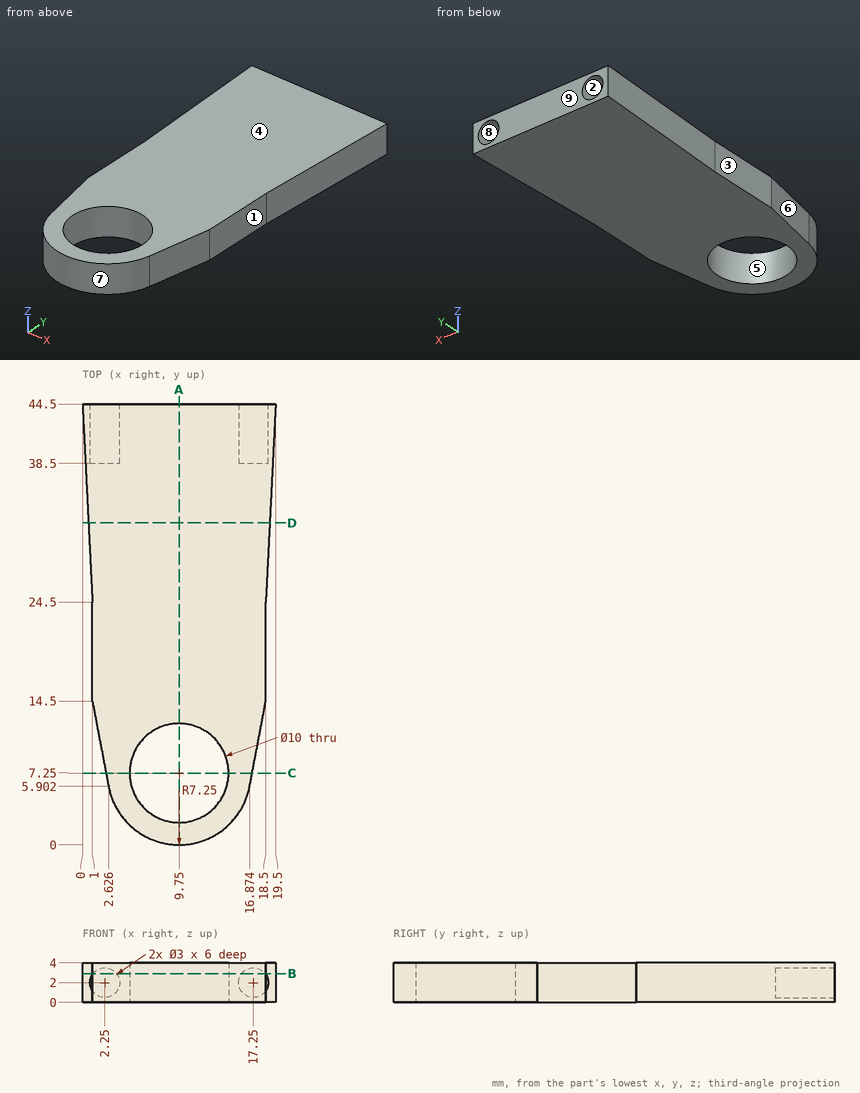
Geometry check sheet. Reference: drawing and pictorial views, mm from the part's lowest x, y, z. A direction names the side the tool comes from. Give positions to 0.01 mm unless a question says otherwise; leave off trailing zeros. Loops run counter-clockwise (first coordinate to the right, second up) from the corner with the lowest first, then second, coordinate; pieces in that order, holes last. Notation, with made-up numbers: M 65,23.25 L 121,23.25 A25 cw 121,61.25 Z; hole C -3,-10.5 d2. An arc over 180 degrees is marked long. One line per question, with ' | ' between items.
Item 1: Depth check by flat-ended pin: P1, Ø2, axis at y = 18, z = 1.5, coming from the -X side; P2, Ø1.2, axis at y = 18.5, z = 2.5, coming from the +X side; P3, Ø1.8, axis at x = 17.25, z = 2, coming from the +Y side. Enter the tip coordinate at first touch or a pass-through.
Completed:
P1: stops at x = 1 | P2: stops at x = 18.5 | P3: stops at y = 38.5
Item 2: Section check D-D, the plane y = 32.5. Record the cut outline in (x, z), plus the area to 3 significant figures.
Completed:
outline: M 0.6,0 L 18.9,0 L 18.9,4 L 0.6,4 Z | area: 73.2 mm^2
Item 3: Draft check along X on the marked faces 6, 7, 8 and 9. Enter one of: +X half, -X half, draft (parallel to the pull), parting line (faces both ways), or undercut.
Completed:
face 6: -X half | face 7: parting line | face 8: undercut | face 9: draft
Item 4: Tool access check on the marked faces 1, 2, 3, 4 and 5. Record the directions out of +Z, -Z, +X, -X, +Y, -Y that give a thin tool (end or side, any length) a straight path to the whole face; none if there is none.
Completed:
face 1: +Z, -Z, +X, -Y | face 2: +Y | face 3: +Z, -Z, -X, -Y | face 4: +Z, +X, -X, +Y, -Y | face 5: +Z, -Z
Item 5: Thickness scan on line 1 (Z direction, x = 2.25, y = 41.15); line 2 (Y direction, x = 9.5, z = 0.55) (1 decimal); line 3 (Y direction, x = 7, z = 1.65) (1 decimal). Record the ranges inside material, lowest first. Write a range as [from, to].
Completed:
line 1: z = [0, 0.5], [3.5, 4] | line 2: y = [0, 2.3], [12.2, 44.5] | line 3: y = [0.5, 3.1], [11.4, 44.5]
Item 6: Section check C-C, the plane y = 7.25. Record the cut outline in (x, z).
Completed:
outline: M 2.37,0 L 4.75,0 L 4.75,4 L 2.37,4 Z; M 14.75,0 L 17.13,0 L 17.13,4 L 14.75,4 Z
Item 7: Section check A-A, the plane x = 9.75. Record the cut outline in (y, z), plus the area to 3 significant figures.
Completed:
outline: M 0,0 L 2.25,0 L 2.25,4 L 0,4 Z; M 12.25,0 L 44.5,0 L 44.5,4 L 12.25,4 Z | area: 138 mm^2
Item 8: Section check B-B, the plane z = 2.9. Record the cut outline in (x, y).
Completed:
outline: M 0,44.5 L 1,24.5 L 1,14.5 L 2.63,5.9 A7.25 ccw 16.87,5.9 L 18.5,14.5 L 18.5,24.5 L 19.5,44.5 L 18.45,44.5 L 18.45,38.5 L 16.05,38.5 L 16.05,44.5 L 3.45,44.5 L 3.45,38.5 L 1.05,38.5 L 1.05,44.5 Z; hole C 9.75,7.25 d10
